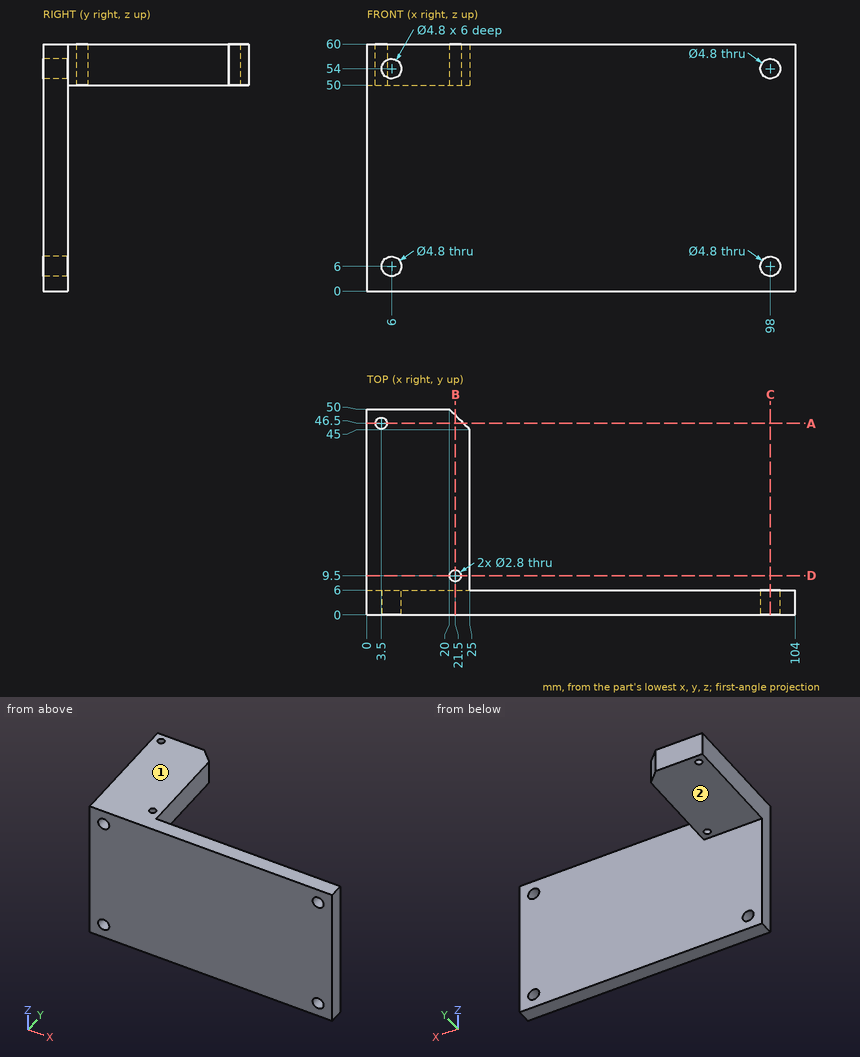
Check sheet for the drawn part. Datum: minimum x, y, z corner. Units: mm. A direction names the side the tool comes from. Round coordinates to 2 decimals unless told otherwise and drop trailing zeros. Write each loop counter-clockwise with the first axis right and the second up, starting at its lowest first coordinate (ties: lowest second). Pieces come first, ordered by that corner, then holes. Notation, with made-up numbers: (-12.5, -14) -> (45.5, -14) arc R34 ccw to (45.5, 17) -> close; hole circle Ø3 at (85.25, 51.25). An arc over 180 degrees is marked (long way). One line per item, written item: value. Start each with the question number.
(1) Access from +Z, -Z, +X, -X, +Y, -Y to the whole of each face (thin tool, end or side, straight path). Record for the marked faces 1 and 2.
(2) Cross-section at A-A, the plane y = 46.5. Record the cut outline in (x, z).
(3) Cross-section at C-C, the plane x = 98. Record the cut outline in (y, z), and give its area (3 significant figures).
(4) Scan lines: line 1 (X direction, y = 1.75, z = 6); line 2 (Z direction, x = 98, y = 1.85); line 3 (Y direction, x = 19.5, z = 36.5). Record each from-to range of solid material in increasing order. Write a range as [from, to].
(5) Go/stop test with flat-tipped pins: pin 1 Ø4 at (x, z) = (41, 7.5) entering from +Y; pin 2 Ø1.7 at (x, y) = (3.5, 46.5) entering from +Z (3 decimals); pin 3 Ø8 at (x, y) = (25.5, 20.5) entering from -Z; pin 4 Ø11 at (y, z) = (33.5, 54) entering from +X. Record where each tip stops, or that it passes through.
(6) Cross-section at B-B, the plane x = 21.5. Record the cut outline in (y, z).
(7) Cross-section at D-D, the plane y = 9.5. Record the cut outline in (x, z), and give its area (3 significant figures).
Answer:
1. face 1: +Z, +X, -X, +Y, -Y
1. face 2: -Z, +X, -X, +Y
2. outline: (0, 50) -> (2.1, 50) -> (2.1, 60) -> (0, 60) -> close; (4.9, 50) -> (23.5, 50) -> (23.5, 60) -> (4.9, 60) -> close
3. outline: (0, 0) -> (6, 0) -> (6, 3.6) -> (0, 3.6) -> close; (0, 8.4) -> (6, 8.4) -> (6, 51.6) -> (0, 51.6) -> close; (0, 56.4) -> (6, 56.4) -> (6, 60) -> (0, 60) -> close
3. area: 302 mm²
4. line 1: [0, 3.6], [8.4, 95.6], [100.4, 104]
4. line 2: [0, 3.6], [8.4, 51.6], [56.4, 60]
4. line 3: [0, 6]
5. pin 1: y = 6
5. pin 2: through
5. pin 3: z = 50
5. pin 4: x = 25
6. outline: (0, 0) -> (6, 0) -> (6, 50) -> (8.1, 50) -> (8.1, 60) -> (0, 60) -> close; (10.9, 50) -> (48.5, 50) -> (48.5, 60) -> (10.9, 60) -> close
7. outline: (0, 50) -> (20.1, 50) -> (20.1, 60) -> (0, 60) -> close; (22.9, 50) -> (25, 50) -> (25, 60) -> (22.9, 60) -> close
7. area: 222 mm²
